The model under review builds one solid part; all positions refer to its coordinate system, in mm. Give positions to 0.01 mm unless a question says otherwise; leave off trailing zeros. Loops run counter-clockwise (first coordinate to the right, second up) from the corner with the lowest first, then second, coordinate; pieces in that order, holes last. Notation, with made-up numbers: (20.25, -23) - (74.25, -23) arc R35 ccw to (74.25, 11) - close; hole circle Ø11 at (-8.5, 48). An arc over 180 degrees is marked (long way). Return JSON: item names as keys, results as strings. Group by question number.
```python
from build123d import *

# Parameters (mm, degrees)
SKETCH1_R           = 1.5
BOSS_EXTRUDE1_DEPTH = 3.175


with BuildPart() as part:
    # Sketch1 → Boss-Extrude1 (new body)
    with BuildSketch(Plane(origin=(0, 3.175, 0), x_dir=(1, 0, 0), z_dir=(0, 1, 0))):
        with BuildLine():
            Line((93.595966692, -79), (134.104033308, -79))
            ThreePointArc((134.104033308, -79), (136.604033308, -79.317541634), (138.945262491, -80.25))
            ThreePointArc((138.945262491, -80.25), (141.85, -81), (144.754737509, -80.25))
            ThreePointArc((144.754737509, -80.25), (147.095966692, -79.317541634), (149.595966692, -79))
            Line((149.595966692, -79), (155.7, -79))
            ThreePointArc((155.7, -79), (157.821320344, -78.121320344), (158.7, -76))
            Line((158.7, -76), (158.7, 76))
            ThreePointArc((158.7, 76), (157.821320344, 78.121320344), (155.7, 79))
            Line((155.7, 79), (149.595966692, 79))
            ThreePointArc((149.595966692, 79), (147.095966692, 79.317541634), (144.754737509, 80.25))
            ThreePointArc((144.754737509, 80.25), (141.85, 81), (138.945262491, 80.25))
            ThreePointArc((138.945262491, 80.25), (136.604033308, 79.317541634), (134.104033308, 79))
            Line((134.104033308, 79), (93.595966692, 79))
            ThreePointArc((93.595966692, 79), (91.095966692, 79.317541635), (88.754737509, 80.25))
            ThreePointArc((88.754737509, 80.25), (85.848773537, 80.999999875), (82.943116423, 80.248812044))
            ThreePointArc((82.943116423, 80.248812044), (80.721943339, 79.347140385), (78.350000001, 79))
            ThreePointArc((78.350000001, 79), (76.228679657, 79.878679657), (75.35, 82))
            Line((75.35, 82), (75.35, 141))
            ThreePointArc((75.35, 141), (74.471320344, 143.121320344), (72.35, 144))
            Line((72.35, 144), (61.495966692, 144))
            ThreePointArc((61.495966692, 144), (58.995966692, 144.317541635), (56.65473751, 145.25))
            ThreePointArc((56.65473751, 145.25), (53.75, 146), (50.845262491, 145.25))
            ThreePointArc((50.845262491, 145.25), (48.504033308, 144.317541635), (46.004033308, 144))
            Line((46.004033308, 144), (-46.004033308, 144))
            ThreePointArc((-46.004033308, 144), (-48.504033308, 144.317541635), (-50.84526249, 145.25))
            ThreePointArc((-50.84526249, 145.25), (-53.75, 146), (-56.654737509, 145.25))
            ThreePointArc((-56.654737509, 145.25), (-58.995966692, 144.317541635), (-61.495966692, 144))
            Line((-61.495966692, 144), (-72.35, 144))
            ThreePointArc((-72.35, 144), (-74.471320344, 143.121320344), (-75.35, 141))
            Line((-75.35, 141), (-75.35, 82))
            ThreePointArc((-75.35, 82), (-76.228679657, 79.878679655), (-78.350000003, 79))
            ThreePointArc((-78.350000003, 79), (-80.72194334, 79.347140385), (-82.943116423, 80.248812044))
            ThreePointArc((-82.943116423, 80.248812044), (-85.848773537, 80.999999874), (-88.754737509, 80.25))
            ThreePointArc((-88.754737509, 80.25), (-91.095966692, 79.317541634), (-93.595966692, 79))
            Line((-93.595966692, 79), (-134.104033308, 79))
            ThreePointArc((-134.104033308, 79), (-136.604033308, 79.317541634), (-138.945262491, 80.25))
            ThreePointArc((-138.945262491, 80.25), (-141.85, 81), (-144.754737509, 80.25))
            ThreePointArc((-144.754737509, 80.25), (-147.095966692, 79.317541634), (-149.595966692, 79))
            Line((-149.595966692, 79), (-155.7, 79))
            ThreePointArc((-155.7, 79), (-157.821320344, 78.121320344), (-158.7, 76))
            Line((-158.7, 76), (-158.7, -76))
            ThreePointArc((-158.7, -76), (-157.821320344, -78.121320344), (-155.7, -79))
            Line((-155.7, -79), (-149.595966692, -79))
            ThreePointArc((-149.595966692, -79), (-147.095966692, -79.317541634), (-144.754737509, -80.25))
            ThreePointArc((-144.754737509, -80.25), (-141.85, -81), (-138.945262491, -80.25))
            ThreePointArc((-138.945262491, -80.25), (-136.604033308, -79.317541634), (-134.104033308, -79))
            Line((-134.104033308, -79), (-93.595966692, -79))
            ThreePointArc((-93.595966692, -79), (-91.095966692, -79.317541634), (-88.754737509, -80.25))
            ThreePointArc((-88.754737509, -80.25), (-85.848773537, -80.999999874), (-82.943116423, -80.248812044))
            ThreePointArc((-82.943116423, -80.248812044), (-80.721943339, -79.347140385), (-78.350000001, -79))
            ThreePointArc((-78.350000001, -79), (-76.228679657, -79.878679656), (-75.35, -82))
            Line((-75.35, -82), (-75.35, -141))
            ThreePointArc((-75.35, -141), (-74.471320344, -143.121320343), (-72.35, -144))
            Line((-72.35, -144), (-61.495966692, -144))
            ThreePointArc((-61.495966692, -144), (-58.995966692, -144.317541634), (-56.654737509, -145.25))
            ThreePointArc((-56.654737509, -145.25), (-53.75, -145.999999999), (-50.84526249, -145.25))
            ThreePointArc((-50.84526249, -145.25), (-48.504033308, -144.317541634), (-46.004033308, -144))
            Line((-46.004033308, -144), (46.004033308, -144))
            ThreePointArc((46.004033308, -144), (48.504033308, -144.317541634), (50.845262491, -145.25))
            ThreePointArc((50.845262491, -145.25), (53.75, -145.999999999), (56.65473751, -145.25))
            ThreePointArc((56.65473751, -145.25), (58.995966692, -144.317541634), (61.495966692, -144))
            Line((61.495966692, -144), (72.35, -144))
            ThreePointArc((72.35, -144), (74.471320344, -143.121320343), (75.35, -141))
            Line((75.35, -141), (75.35, -82))
            ThreePointArc((75.35, -82), (76.228679656, -79.878679656), (78.35, -79))
            ThreePointArc((78.35, -79), (80.721943339, -79.347140384), (82.943116423, -80.248812044))
            ThreePointArc((82.943116423, -80.248812044), (85.848773537, -80.999999874), (88.754737509, -80.25))
            ThreePointArc((88.754737509, -80.25), (91.095966692, -79.317541634), (93.595966692, -79))
        make_face()
        with Locations((141.85, -75)):
            Circle(SKETCH1_R, mode=Mode.SUBTRACT)
        with Locations((85.85, -75)):
            Circle(SKETCH1_R, mode=Mode.SUBTRACT)
        with Locations((53.75, -140)):
            Circle(SKETCH1_R, mode=Mode.SUBTRACT)
        with Locations((-53.75, -140)):
            Circle(SKETCH1_R, mode=Mode.SUBTRACT)
        with Locations((-85.85, -75)):
            Circle(SKETCH1_R, mode=Mode.SUBTRACT)
        with Locations((-141.85, -75)):
            Circle(SKETCH1_R, mode=Mode.SUBTRACT)
        with Locations((141.85, 75)):
            Circle(SKETCH1_R, mode=Mode.SUBTRACT)
        with Locations((85.849999999, 75)):
            Circle(SKETCH1_R, mode=Mode.SUBTRACT)
        with Locations((53.75, 140)):
            Circle(SKETCH1_R, mode=Mode.SUBTRACT)
        with Locations((-53.75, 140)):
            Circle(SKETCH1_R, mode=Mode.SUBTRACT)
        with Locations((-85.85, 75)):
            Circle(SKETCH1_R, mode=Mode.SUBTRACT)
        with Locations((-141.85, 75)):
            Circle(SKETCH1_R, mode=Mode.SUBTRACT)
        with Locations((-35.9, 124)):
            Circle(SKETCH1_R, mode=Mode.SUBTRACT)
        with Locations((35.9, 124)):
            Circle(SKETCH1_R, mode=Mode.SUBTRACT)
        with Locations((-35.9, -11.5)):
            Circle(SKETCH1_R, mode=Mode.SUBTRACT)
        with Locations((35.9, -11.5)):
            Circle(SKETCH1_R, mode=Mode.SUBTRACT)
    extrude(amount=-BOSS_EXTRUDE1_DEPTH)


solid = part.part
```
1) We need section A-A, the plane y = 1.45. Count the separate pieces of the cut face and the enclosed holes in it, plus the area to 3 significant figures.
2) We need section B-B, the plane z = 121. Write out the cut boundary in (x, y) (3 decimals), plus the area to 3 significant figures.
3) To check wall thickness, follow line 1 (X direction, y = 2.1, z = 11.5); line 2 (Z direction, x = -85.85, y = 0.8); line 3 (X direction, y = 0.75, z = 75). State the ranges of each line that lie inside material, in increasing order.
4) For pin 1 Ø1.6 at (y, z) = (1, 115) entering from +X; pin 2 Ø1.6 at (y, z) = (2, 108) entering from -X; pin 3 Ø1.6 at (x, y) = (-4.5, 2) entering from -Z; pin 4 Ø1.8 at (x, z) = (-35.9, 11.5) entering from -Y, all flat-tipped, find the tip position at first contact; note any pin that passes through.
Findings:
{
 "1": {"separate pieces": "1", "enclosed holes": "16", "area": "69,800 mm^2"},
 "2": {"outline": "(-75.35, 0) - (75.35, 0) - (75.35, 3.175) - (-75.35, 3.175) - close", "area": "478 mm^2"},
 "3": {"line 1": "x = -158.7 to -37.4, -34.4 to 34.4, 37.4 to 158.7", "line 2": "z = -81 to -76.5, -73.5 to 73.5, 76.5 to 81", "line 3": "x = -158.7 to -143.35, -140.35 to -87.35, -84.35 to 84.35, 87.35 to 140.35, 143.35 to 158.7"},
 "4": {"pin 1": "stops at x = 75.35", "pin 2": "stops at x = -75.35", "pin 3": "stops at z = -144", "pin 4": "passes through"}
}
